Study the drawing (mm; zero at the part's minimum x, y, z) and answer. A direction names the side the tool comes from. Give positions to 0.01 mm unless a question says otherwise; leave off trailing zeros. Order: outer loops, then holes, each group sorted by start corner. A loop starts at its lowest first (then second) coordinate and runs counter-clockwise, first axis right, second up. Notation, with made-up numbers: (-35.5, 46.5) - (3.5, 46.5) arc R10 ccw to (3.5, 63.5) - close; hole circle Ø4 at (35, -16). An arc over 180 degrees is marked (long way). Write each question's results on one line, items separated by ' | '. Start each with the question number.
Q1. Find section C-C on x = 14. Count the separate pieces of the cut face and the enclosed holes in it, and give its area (3 significant figures).
Q2. For a pull along Y with two mould halves and no side action, classify the marked faces 1, 2 and 3 as +Y half, -Y half, draft (parallel to the pull), parting line (faces both ways), or undercut.
Q3. Find section B-B on y = 15. Give the vertices of the cut face in (x, z) (1 decimal).
Q4. A tool of negligible diameter and unlimited length cuts with its end or side. For the marked faces 4, 5 and 6, from which of +Z, -Z, +X, -X, +Y, -Y can it reach the whole face along a straight path? Write none if from no direction.
Q5. Find the intervals of material crossed by line 1 along Y through (x, z) = (16.5, 20) (1 decimal); line 2 along Z through (x, y) = (16.5, 24.5); line 3 along Y through (x, z) = (16, 17.5) (1 decimal), in increasing order. Write a range as from..to.
Q6. Flat-ended cylindrical pins translate along their axes: P1, Ø6, axis at x = 4.17, y = 8.75, coming from the +Z side; P2, Ø3, axis at y = 7.5, z = 9.5, coming from the -X side; P3, Ø5, axis at x = 7.5, z = 6.5, coming from the +Y side. Find the tip coordinate at first contact, or state that the pin passes through.
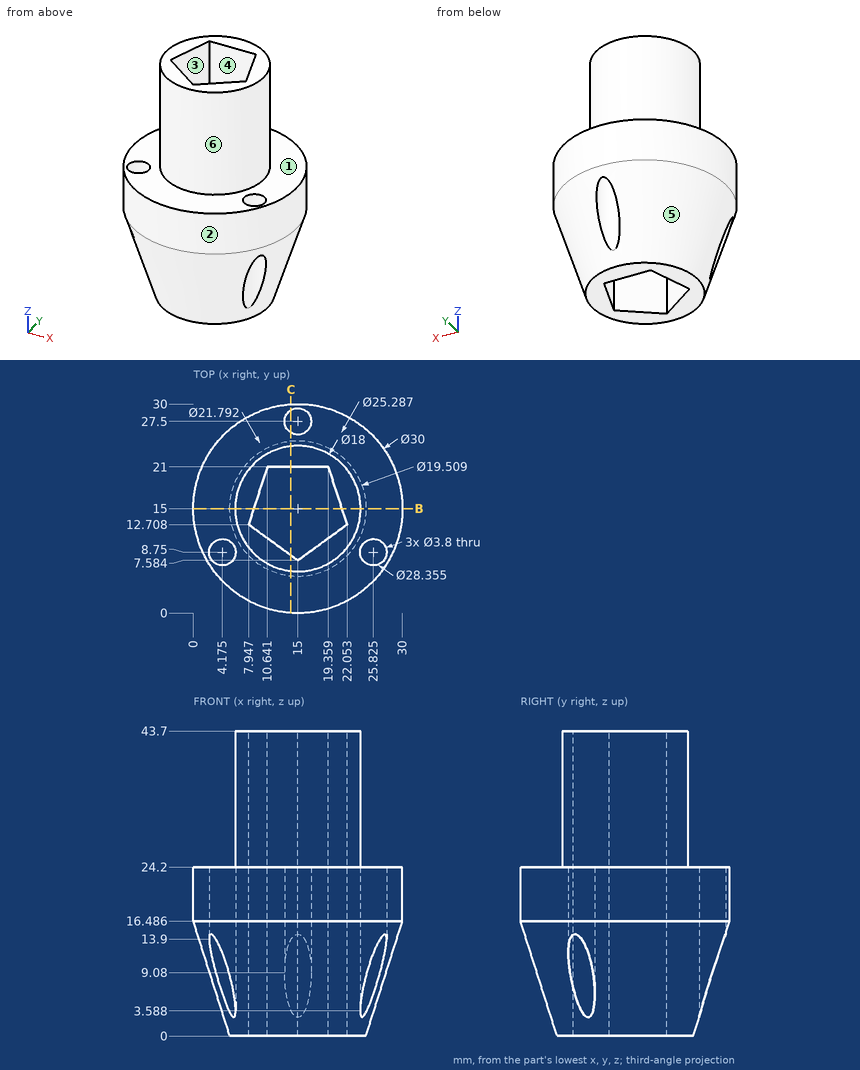
Working result:
1) separate pieces: 3 | enclosed holes: 0 | area: 382 mm²
2) face 1: draft | face 2: parting line | face 3: undercut
3) outline: (0, 16.5) - (5.2, 0) - (8.7, 0) - (8.7, 43.7) - (6, 43.7) - (6, 24.2) - (0, 24.2) - close; (21.3, 0) - (24.8, 0) - (30, 16.5) - (30, 24.2) - (24, 24.2) - (24, 43.7) - (21.3, 43.7) - close
4) face 4: +Z, -Z | face 5: -Z | face 6: +Z
5) line 1: 0.1..8.7, 21..26.3, 28.7..29.9 | line 2: 0..24.2 | line 3: 0..8.3, 21..25.9, 29.1..30
6) P1: z = 24.2 | P2: x = 4.57 | P3: y = 26
